Verification items for the finished model (mm, model axes). A direction names the side the tool comes from. Give positions to 0.01 mm unless a question says otherwise; leave off trailing zeros. Order: outer loops, then holes, each group sorted by start corner. A loop starts at its lowest first (then second) coordinate and runs counter-clockwise, first axis right, second up. Notation, with made-up numbers: (3.5, -15) -> (51.5, -15) arc R18 ccw to (51.5, 17) -> close; hole circle Ø7 at (16.5, 34.5). An arc over 180 degrees is marked (long way). Return JSON: item names as keys, results as strings. Group by question number.
(1) Tool access check on faces 1 (the face through (1.15, 35.27, -7.79)), 2 (the face through (4, 110, -7)), 3 (the face through (-4, -110, -7)), 4 (the face through (-7.79, 35.36, 0.9)). Record the directions out of +Z, -Z, +X, -X, +Y, -Y that give a thin tool (end or side, any length) a straight path to the whole face; none if there is none.
(2) Cross-section at A-A on y = -24.5. Enter the section's corners in (x, z), then the cut area to 3 significant figures.
(3) Thickness scan on line 1 along Y through (x, z) = (0, -7.95); line 2 along X through (y, z) = (-80.5, -7.85); line 3 along X through (y, z) = (48, -0.5). Record the ranges inside material, lowest first.
(4) Release check for a two-part mould opening along Z. For faces 5 (the face through (1.172, 1.537, -8.923)), 6 (the face through (0.2, -32.02, -5.51)), 7 (the face through (0, 118, 0)), 8 (the face through (-5.51, 32.98, -0.2)) record: pulls with the +Z half, pulls with the -Z half, needs draft (parallel to the pull), parting line crosses it, or undercut.
(5) Depth check by flat-ended pin: pin 1 Ø5.5 at (x, y) = (0, -80.5) entering from -Z; pin 2 Ø5 at (y, z) = (32.5, 0) entering from -X; pin 3 Ø8 at (x, y) = (-5.5, -33) entering from +Z. Enter the tip coordinate at first touch or a pass-through.
from build123d import *

# Parameters (mm, degrees)
CHAMFER_1_SIZE                 = 0.5
HOLE_WIZARD_6_0_6_4_AT_2_COUNT = 2
HOLE_WIZARD_6_0_6_4_AT_2_PITCH = 65
HOLE_WIZARD_6_0_6_4_AT_3_COUNT = 2
HOLE_WIZARD_6_0_6_4_AT_3_PITCH = 113
HOLE_WIZARD_6_0_6_4_AT_4_COUNT = 2
HOLE_WIZARD_6_0_6_4_AT_4_PITCH = 48
PATTERN_CIRCULAR_1_COUNT       = 4
CHAMFER_2_SIZE                 = 0.2


with BuildPart() as part:
    # 草图1 → 旋转1 (revolve)
    with BuildSketch(Plane.XY):
        Polygon((0, 118), (0, -118), (-7.5, -118), (-7.5, -110), (-9, -110), (-9, 110), (-7.5, 110), (-7.5, 118), align=None)
    revolve(axis=Axis((0, 118, 0), (0, -1, 0)))

    # 倒角1
    chamfer_1_edges = [part.edges().sort_by_distance(p)[0] for p in [
        (7.5, 118, 0),
        (7.5, -118, 0),
    ]]
    chamfer(chamfer_1_edges, length=CHAMFER_1_SIZE)

    # 草图3 → Ø6.0 (6) 直径孔4 (revolve, cut)
    with BuildSketch(Plane(origin=(0, -32.5, -9), x_dir=(0, 1, 0), z_dir=(1, 0, 0))):
        Polygon((0, 0), (0, 3.802581857), (3, 2), (3, 0), align=None)
    hole_wizard_6_0_6_4 = revolve(axis=Axis((0, -32.5, -15.35), (0, 0, 1)), mode=Mode.SUBTRACT)

    # Ø6.0 (6) 直径孔4 at 2: Ø6.0 (6) 直径孔4 ×2
    with Locations(*[(0, i * HOLE_WIZARD_6_0_6_4_AT_2_PITCH, 0) for i in range(1, HOLE_WIZARD_6_0_6_4_AT_2_COUNT)]):
        add(hole_wizard_6_0_6_4, mode=Mode.SUBTRACT)

    # Ø6.0 (6) 直径孔4 at 3: Ø6.0 (6) 直径孔4 ×2
    with Locations(*[(0, i * HOLE_WIZARD_6_0_6_4_AT_3_PITCH, 0) for i in range(1, HOLE_WIZARD_6_0_6_4_AT_3_COUNT)]):
        add(hole_wizard_6_0_6_4, mode=Mode.SUBTRACT)

    # Ø6.0 (6) 直径孔4 at 4: Ø6.0 (6) 直径孔4 ×2
    with Locations(*[(0, -i * HOLE_WIZARD_6_0_6_4_AT_4_PITCH, 0) for i in range(1, HOLE_WIZARD_6_0_6_4_AT_4_COUNT)]):
        add(hole_wizard_6_0_6_4, mode=Mode.SUBTRACT)

    # 阵列(圆周)1: Ø6.0 (6) 直径孔4 ×4 about axis, 2 skipped
    pattern_circular_1_axis = Axis((0, 118, 0), (0, 1, 0))
    add([hole_wizard_6_0_6_4.rotate(pattern_circular_1_axis, i * 360 / PATTERN_CIRCULAR_1_COUNT) for i in range(1, PATTERN_CIRCULAR_1_COUNT) if i not in (2, 3)], mode=Mode.SUBTRACT)

    # 阵列(圆周)1 copy 1 sketch → 阵列(圆周)1 copy 1 (revolve, cut)
    with BuildSketch(Plane(origin=(-9, 32.5, 0), x_dir=(0, 1, 0), z_dir=(0, 0, -1))):
        Polygon((0, 0), (0, 3.802581857), (3, 2), (3, 0), align=None)
    revolve(axis=Axis((-15.35, 32.5, 0), (1, 0, 0)), mode=Mode.SUBTRACT)

    # 阵列(圆周)1 copy 2 sketch → 阵列(圆周)1 copy 2 (revolve, cut)
    with BuildSketch(Plane(origin=(-9, 80.5, 0), x_dir=(0, 1, 0), z_dir=(0, 0, -1))):
        Polygon((0, 0), (0, 3.802581857), (3, 2), (3, 0), align=None)
    revolve(axis=Axis((-15.35, 80.5, 0), (1, 0, 0)), mode=Mode.SUBTRACT)

    # 阵列(圆周)1 copy 3 sketch → 阵列(圆周)1 copy 3 (revolve, cut)
    with BuildSketch(Plane(origin=(-9, -80.5, 0), x_dir=(0, 1, 0), z_dir=(0, 0, -1))):
        Polygon((0, 0), (0, 3.802581857), (3, 2), (3, 0), align=None)
    revolve(axis=Axis((-15.35, -80.5, 0), (1, 0, 0)), mode=Mode.SUBTRACT)

    # 倒角2
    chamfer_2_edges = [part.edges().sort_by_distance(p)[0] for p in [
        (9, 110, 0),
        (9, -110, 0),
    ]]
    chamfer(chamfer_2_edges, length=CHAMFER_2_SIZE)


solid = part.part
Verdict:
{
 "1": {"face 1": "-Z", "face 2": "+Y", "face 3": "-Y", "face 4": "-X"},
 "2": {"outline": "circle Ø18 at (0, 0)", "area": "254 mm²"},
 "3": {"line 1": "-110 to -83.5, -77.5 to -35.5, -29.5 to 29.5, 35.5 to 77.5, 83.5 to 110", "line 2": "-4.4 to -3, 3 to 4.4", "line 3": "-8.99 to 8.99"},
 "4": {"face 5": "parting line crosses it", "face 6": "pulls with the -Z half", "face 7": "needs draft", "face 8": "undercut"},
 "5": {"pin 1": "z = -6.85", "pin 2": "x = -6.7", "pin 3": "z = 8.87"}
}
